from build123d import *

# Parameters (mm, degrees)
BOSS_EXTRUDE1_DEPTH = 6.35
SKETCH2_R           = 3.175
CUT_EXTRUDE1_DEPTH  = 5.588
BOSS_EXTRUDE2_DEPTH = 0.762
SKETCH4_R           = 1.016
CUT_EXTRUDE2_DEPTH  = 7.35
CUT_EXTRUDE3_DEPTH  = 30.21
CUT_EXTRUDE4_DEPTH  = 25.384


with BuildPart() as part:
    # Sketch1 → Boss-Extrude1 (new body)
    with BuildSketch(Plane(origin=(0, 0, 0), x_dir=(1, 0, 0), z_dir=(0, 1, 0))):
        Polygon((77.849076972, 47.983166812), (28.319076972, 47.983166812), (28.319076972, 43.157166812), (23.239076972, 43.157166812), (23.239076972, 23.599166812), (28.319076972, 23.599166812), (28.319076972, 18.773166812), (77.849076972, 18.773166812), align=None)
    extrude(amount=-BOSS_EXTRUDE1_DEPTH)

    # Sketch2 → Cut-Extrude1 (cut)
    with BuildSketch(Plane(origin=(0, 0, 0), x_dir=(1, 0, 0), z_dir=(0, 1, 0))):
        with Locations((42.143084751, 41.34242402)):
            Circle(SKETCH2_R)
        with Locations((32.069218962, 30.263111699)):
            Circle(SKETCH2_R)
        with Locations((40.161790785, 26.014596512)):
            Circle(SKETCH2_R)
        with Locations((57.943162236, 33.942485163)):
            Circle(SKETCH2_R)
        with Locations((57.943162236, 24.036485163)):
            Circle(SKETCH2_R)
        with Locations((69.631305355, 35.731766034)):
            Circle(SKETCH2_R)
        with BuildLine():
            Line((46.919562236, 30.970685163), (46.919562236, 27.008285163))
            ThreePointArc((46.919562236, 27.008285163), (48.037162236, 20.861485163), (49.154762236, 27.008285163))
            Line((49.154762236, 27.008285163), (49.154762236, 30.970685163))
            ThreePointArc((49.154762236, 30.970685163), (48.037162236, 37.117485163), (46.919562236, 30.970685163))
        make_face()
    extrude(amount=-CUT_EXTRUDE1_DEPTH, mode=Mode.SUBTRACT)

    # Sketch3 → Boss-Extrude2 (add)
    with BuildSketch(Plane(origin=(0, 0, 0), x_dir=(1, 0, 0), z_dir=(0, 1, 0))):
        Polygon((77.849076972, 33.759166812), (75.055076972, 32.362166812), (75.055076972, 31.092166812), (77.849076972, 29.695166812), align=None)
    extrude(amount=BOSS_EXTRUDE2_DEPTH)

    # Sketch4 → Cut-Extrude2 (cut, through all)
    with BuildSketch(Plane(origin=(0, 0, 0), x_dir=(1, 0, 0), z_dir=(0, 1, 0))):
        with Locations((69.631305355, 35.731766034)):
            Circle(SKETCH4_R)
        with Locations((40.161790785, 26.014596512)):
            Circle(SKETCH4_R)
    extrude(amount=-CUT_EXTRUDE2_DEPTH, mode=Mode.SUBTRACT)

    # Sketch5 → Cut-Extrude3 (cut, through all)
    with BuildSketch(Plane.XY.offset(-18.773166812)):
        Polygon((77.849076972, -3.81), (76.579076972, -6.35), (77.849076972, -6.35), align=None)
    extrude(amount=-CUT_EXTRUDE3_DEPTH, mode=Mode.SUBTRACT)

    # Sketch6 → Cut-Extrude4 (cut, through all)
    with BuildSketch(Plane.XY.offset(-23.599166812)):
        Polygon((25.271076972, -6.35), (23.239076972, -2.032), (23.239076972, -6.35), align=None)
    extrude(amount=-CUT_EXTRUDE4_DEPTH, mode=Mode.SUBTRACT)


solid = part.part
Geometry: final body of the model. Coordinates: model frame, mm. A direction names the side the tool comes from. Round coordinates to 2 decimals unless told otherwise and drop trailing zeros. Order: outer loops, then holes, each group sorted by start corner. A loop starts at its lowest first (then second) coordinate and runs counter-clockwise, first axis right, second up. Notation, with made-up numbers: (-21.75, 2.25) -> (16.25, 2.25) arc R22 ccw to (16.25, 27.25) -> close; hole circle Ø7 at (15.5, 67). An arc over 180 degrees is marked (long way). Put each result on its own line as item: value. Start each with the question number.
Q1. Section C-C on z = -22.25. Return the cut outline in (x, y), and give its area (3 significant figures).
Q2. Reachability of faces 5 (the flat face through (28.319, -3, -21)), 6 (the cylindrical face through (47.914, -2.755, -20.864)), 7 (the cylindrical face through (40.71, -5.96, -26.87)) from +Z, -Z, +X, -X, +Y, -Y: full face, straight path, thin tool, end or side. Return the list, or none.
Q3. First-contact query: pin 1 (2 mm diameter, centred on y = -5.5, z = -26, fed in from -X); pin 2 (1 mm diameter, centred on y = -3.5, z = -29.5, fed in from -X); pin 3 (2.5 mm diameter, centred on y = -4, z = -21.5, fed in from -X). Flat tips, straight axial feed; report the tip coordinate or a pass-through.
Q4. Section B-B on y = -4.75. Return the cut outline in (x, z) (3 decimals).
Q5. Section D-D on x = 29.5. Return the cut outline in (y, z).
Q6. Section A-A on x = 58. Return the cut outline in (y, z), and give its area (3 significant figures).
Q7. Line query: probe 1 along X at (y, z) = (-2.25, -23.5); probe 2 along Z at (x, y) = (49.5, -3.25); probe 3 along X at (y, z) = (-4.5, -30.5). Output: solid intervals per line, ascending.
Q8. Pull-direction query (Z, two-part tool) for faces 1 (the flat face through (76.47, 0.38, -33.07)), 2 (the flat face through (26, -3, -23.599)), 3 (the cylindrical face through (43.095, -2.755, -24.799)), 4 (the flat face through (24.27, -4.22, -33.24)); classes: +Z half, -Z half, draft (parallel to the pull), parting line (faces both ways), or undercut.
Ans:
1. outline: (28.32, -6.35) -> (76.58, -6.35) -> (77.85, -3.81) -> (77.85, 0) -> (60.57, 0) -> (60.57, -5.59) -> (55.32, -5.59) -> (55.32, 0) -> (50.66, 0) -> (50.66, -5.59) -> (45.41, -5.59) -> (45.41, 0) -> (28.32, 0) -> close
1. area: 254 mm2
2. face 5: +Z, -X, +Y, -Y
2. face 6: +Y
2. face 7: +Y, -Y
3. pin 1: stops at x = 24.4
3. pin 2: stops at x = 23.69
3. pin 3: stops at x = 28.32
4. outline: (24.518, -43.157) -> (28.319, -43.157) -> (28.319, -47.983) -> (77.379, -47.983) -> (77.379, -18.773) -> (28.319, -18.773) -> (28.319, -23.599) -> (24.518, -23.599) -> close; hole circle Ø6.35 at (32.069, -30.263); hole circle Ø6.35 at (40.162, -26.015); hole circle Ø6.35 at (42.143, -41.342); hole (46.92, -30.971) arc R3.175 ccw (long way) to (49.155, -30.971) -> (49.155, -27.008) arc R3.175 ccw (long way) to (46.92, -27.008) -> close; hole circle Ø6.35 at (57.943, -33.942); hole circle Ø6.35 at (57.943, -24.036); hole circle Ø6.35 at (69.631, -35.732)
5. outline: (-6.35, -47.98) -> (0, -47.98) -> (0, -32.13) -> (-5.59, -32.13) -> (-5.59, -28.4) -> (0, -28.4) -> (0, -18.77) -> (-6.35, -18.77) -> close
6. outline: (-6.35, -47.98) -> (0, -47.98) -> (0, -37.12) -> (-5.59, -37.12) -> (-5.59, -30.77) -> (0, -30.77) -> (0, -27.21) -> (-5.59, -27.21) -> (-5.59, -20.86) -> (0, -20.86) -> (0, -18.77) -> (-6.35, -18.77) -> close
6. area: 115 mm2
7. probe 1: x = 28.32 to 38.22, 42.1 to 44.91, 51.17 to 54.81, 61.07 to 77.85
7. probe 2: z = -47.98 to -36.76, -31.12 to -26.85, -21.22 to -18.77
7. probe 3: x = 24.4 to 28.9, 35.24 to 46.92, 49.15 to 77.5
8. face 1: -Z half
8. face 2: +Z half
8. face 3: undercut
8. face 4: draft
